Could you check a few things on this model? Use its own coordinates, in mm. Face numbers are marked on the shaded views. A direction names the side the tool comes from. Coordinates: 2 decimals unless noted, no trailing zeros. Write each loop counter-clockwise with the first axis right and the second up, starting at its lowest first coordinate (ties: lowest second). Pieces come first, ordered by that corner, then holes.
```python
from build123d import *

# Parameters (mm, degrees)
EXTRUDE_1_DEPTH        = 65
CUT_EXTRUDE_1_DEPTH    = 57.5
SKETCH_4_R             = 1.25
SKETCH_4_W             = 13
SKETCH_4_H             = 28.5
CUT_EXTRUDE_2_DEPTH    = 13
SKETCH_9_W             = 13
SKETCH_9_H             = 38.4
CUT_EXTRUDE_6_DEPTH    = 75.806476324
CUT_EXTRUDE_7_DEPTH    = 18
SKETCH_13_W            = 21
SKETCH_13_H            = 5
CUT_EXTRUDE_10_DEPTH   = 18
CUT_EXTRUDE_8_DEPTH    = 78.086308123
CUT_EXTRUDE_9_DEPTH    = 10
FILLET_1_R             = 4
FILLET_1_OF_MIRROR_3_R = 4
SKETCH_21_W            = 21
SKETCH_21_H            = 14
CUT_EXTRUDE_17_DEPTH   = 8
SKETCH_17_W            = 19.798748342
SKETCH_17_H            = 9
CUT_EXTRUDE_13_DEPTH   = 3
SKETCH_18_W            = 14
SKETCH_18_H            = 18
CUT_EXTRUDE_14_DEPTH   = 5
SKETCH_19_R            = 4
CUT_EXTRUDE_15_DEPTH   = 10
FILLET_6_R             = 2
SKETCH_5_R             = 12
CUT_EXTRUDE_3_DEPTH    = 8
CUT_EXTRUDE_16_DEPTH   = 61.954985592
CUT_EXTRUDE_18_DEPTH   = 25
CUT_EXTRUDE_19_DEPTH   = 20
CUT_EXTRUDE_5_DEPTH    = 76.706738594
CUT_EXTRUDE_20_DEPTH   = 12
FILLET_5_R             = 10


with BuildPart() as part:
    # 草圖1 → 填料-伸長1 (new body)
    with BuildSketch(Plane(origin=(0, 0, 0), x_dir=(1, 0, 0), z_dir=(0, 1, 0))):
        Polygon((0, 0), (24.34, 0), (34.67, -10.33), (34.67, -22.7), (-10.33, -22.7), (-10.33, -10.33), align=None)
    extrude(amount=EXTRUDE_1_DEPTH)

    # 草圖2 → 除料-伸長1 (cut)
    with BuildSketch(Plane(origin=(0, 5, 0), x_dir=(1, 0, 0), z_dir=(0, 1, 0))):
        Polygon((0, 0), (-22.7, -22.7), (-17.043145751, -22.7), (5.656854249, 0), align=None)
    cut_extrude_1 = extrude(amount=CUT_EXTRUDE_1_DEPTH, mode=Mode.SUBTRACT)

    # 鏡射1: 除料-伸長1 across plane
    add(cut_extrude_1.mirror(Plane.ZY.offset(-12.17)), mode=Mode.SUBTRACT)

    # 草圖4 → 除料-伸長2 (cut)
    with BuildSketch(Plane.XY.offset(22.7)):
        with Locations((12.17, 59.36)):
            Circle(SKETCH_4_R)
        with Locations((12.17, 24.36)):
            Circle(SKETCH_4_R)
        with Locations((12.17, 41.86)):
            Rectangle(SKETCH_4_W, SKETCH_4_H)
    extrude(amount=-CUT_EXTRUDE_2_DEPTH, mode=Mode.SUBTRACT)

    # 草圖9 → 除料-伸長6 (cut, through all)
    with BuildSketch(Plane.XY.offset(9.7)):
        with Locations((12.17, 41.86)):
            Rectangle(SKETCH_9_W, SKETCH_9_H)
    extrude(amount=-CUT_EXTRUDE_6_DEPTH, mode=Mode.SUBTRACT)

    # 草圖10 → 除料-伸長7 (cut)
    with BuildSketch(Plane.XZ):
        Polygon((20.67, 3), (3.67, 3), (1.67, 5), (1.67, 10), (22.67, 10), (22.67, 5), align=None)
    extrude(amount=-CUT_EXTRUDE_7_DEPTH, mode=Mode.SUBTRACT)

    # 草圖13 → 除料-伸長10 (cut)
    with BuildSketch(Plane.XZ):
        with Locations((12.17, 12.5)):
            Rectangle(SKETCH_13_W, SKETCH_13_H)
    extrude(amount=-CUT_EXTRUDE_10_DEPTH, mode=Mode.SUBTRACT)

    # 草圖11 → 除料-伸長8 (cut, through all)
    with BuildSketch(Plane.XZ):
        Polygon((-9.55794071, 4.584194914), (-25.114289896, 20.1405441), (-14.849242405, 30.405591591), (0.707106781, 14.849242405), align=None)
    cut_extrude_8 = extrude(amount=-CUT_EXTRUDE_8_DEPTH, mode=Mode.SUBTRACT)

    # 草圖12 → 除料-伸長9 (cut)
    with BuildSketch(Plane.XZ):
        Polygon((-4.242640687, 9.899494937), (-19.798989873, 25.455844123), (-11.313708499, 33.941125497), (4.242640687, 18.384776311), align=None)
    cut_extrude_9 = extrude(amount=-CUT_EXTRUDE_9_DEPTH, mode=Mode.SUBTRACT)

    # 圓角1
    fillet_1_edges = [part.edges().sort_by_distance(p)[0] for p in [
        (-3.218272016, 10, 18.774621202),
    ]]
    fillet(fillet_1_edges, radius=FILLET_1_R)

    # 鏡射3: 除料-伸長8, 除料-伸長9 across plane
    add(cut_extrude_8.mirror(Plane.ZY.offset(-12.17)), mode=Mode.SUBTRACT)
    add(cut_extrude_9.mirror(Plane.ZY.offset(-12.17)), mode=Mode.SUBTRACT)

    # 圓角1 of 鏡射3
    fillet_1_of_mirror_3_edges = [part.edges().sort_by_distance(p)[0] for p in [
        (27.558272016, 10, 18.774621202),
    ]]
    fillet(fillet_1_of_mirror_3_edges, radius=FILLET_1_OF_MIRROR_3_R)

    # 草圖21 → 除料-伸長17 (cut)
    with BuildSketch(Plane(origin=(0, 0, 0), x_dir=(-1, 0, 0), z_dir=(0, 0, -1))):
        with Locations((-12.17, 7)):
            Rectangle(SKETCH_21_W, SKETCH_21_H)
    extrude(amount=-CUT_EXTRUDE_17_DEPTH, mode=Mode.SUBTRACT)

    # 草圖17 → 除料-伸長13 (cut)
    with BuildSketch(Plane(origin=(2.828427125, 0, 2.828427125), x_dir=(-0.7071067811865472, 0, 0.7071067811865479), z_dir=(-0.7071067811865479, 0, -0.7071067811865472))):
        with Locations((11.537637522, 9.5)):
            Rectangle(SKETCH_17_W, SKETCH_17_H)
    extrude(amount=-CUT_EXTRUDE_13_DEPTH, mode=Mode.SUBTRACT)

    # 草圖18 → 除料-伸長14 (cut)
    with BuildSketch(Plane.XY.offset(15)):
        with Locations((12.17, 9)):
            Rectangle(SKETCH_18_W, SKETCH_18_H)
    extrude(amount=CUT_EXTRUDE_14_DEPTH, mode=Mode.SUBTRACT)

    # 草圖19 → 除料-伸長15 (cut)
    with BuildSketch(Plane.XY.offset(22.7)):
        with Locations((12.17, 24.36)):
            Circle(SKETCH_19_R)
    extrude(amount=-CUT_EXTRUDE_15_DEPTH, mode=Mode.SUBTRACT)

    # 圓角6
    fillet_6_edges = [part.edges().sort_by_distance(p)[0] for p in [
        (0.707106781, 39.5, 14.849242405),
        (3.889087297, 10, 18.03122292),
        (1.535533906, 11.171572875, 15.67766953),
        (23.632893219, 39.5, 14.849242405),
        (20.450912703, 10, 18.03122292),
        (22.804466094, 11.171572875, 15.67766953),
    ]]
    fillet(fillet_6_edges, radius=FILLET_6_R)

    # 草圖5 → 除料-伸長3 (cut)
    with BuildSketch(Plane.XY.offset(22.7)):
        with Locations((12.17, 50)):
            Circle(SKETCH_5_R)
    extrude(amount=-CUT_EXTRUDE_3_DEPTH, mode=Mode.SUBTRACT)

    # 草圖20 → 除料-伸長16 (cut, through all)
    with BuildSketch(Plane.XZ.offset(-18)):
        Polygon((4.17, 3.608174593), (-2.121320344, 9.899494937), (1.17918472, 13.2), (4.17, 13.2), align=None)
        Polygon((20.17, 13.2), (23.16081528, 13.2), (26.461320344, 9.899494937), (20.17, 3.608174593), align=None)
    extrude(amount=-CUT_EXTRUDE_16_DEPTH, mode=Mode.SUBTRACT)

    # 草圖22 → 除料-伸長18 (cut)
    with BuildSketch(Plane.XZ.offset(-14)):
        Polygon((1.414213562, 16.263455967), (-3.52233047, 21.2), (3.67, 21.2), (3.67, 18.519242405), align=None)
        Polygon((27.86233047, 21.2), (20.67, 21.2), (20.67, 18.519242405), (22.925786438, 16.263455967), align=None)
    extrude(amount=-CUT_EXTRUDE_18_DEPTH, mode=Mode.SUBTRACT)

    # 草圖23 → 除料-伸長19 (cut)
    with BuildSketch(Plane.XZ.offset(-18)):
        Polygon((4.17, 13.2), (1.17918472, 13.2), (4.17, 16.19081528), align=None)
        Polygon((23.16081528, 13.2), (20.17, 16.19081528), (20.17, 13.2), align=None)
    extrude(amount=-CUT_EXTRUDE_19_DEPTH, mode=Mode.SUBTRACT)

    # 草圖8 → 除料-伸長5 (cut, through all)
    with BuildSketch(Plane.XY.offset(22.7)):
        with BuildLine():
            Line((4.67, 70), (4.67, 73.83732793))
            Line((4.67, 73.83732793), (19.67, 73.83732793))
            Line((19.67, 73.83732793), (19.67, 70))
            ThreePointArc((19.67, 70), (12.17, 62.5), (4.67, 70))
        make_face()
    extrude(amount=-CUT_EXTRUDE_5_DEPTH, mode=Mode.SUBTRACT)

    # 草圖7 → 除料-伸長20 (cut)
    with BuildSketch(Plane.XY.offset(22.7)):
        with BuildLine():
            Line((-2.83, 70), (27.17, 70))
            ThreePointArc((27.17, 70), (12.17, 55), (-2.83, 70))
        make_face()
    extrude(amount=-CUT_EXTRUDE_20_DEPTH, mode=Mode.SUBTRACT)

    # 圓角5
    # the kernel refuses this fillet: 10 mm, written as the material it takes off along each edge
    with BuildSketch(Plane(origin=(3.203430143, 57.975, 14.7), x_dir=(-0.6822618553726185, 0.7311078994946726, 0), z_dir=(0, 0, 1))) as fillet_5_piece_1:
        with BuildLine():
            CenterArc((7.130730412, 9.839819243), FILLET_5_R, 209.862696675, 49.868396236)
            ThreePointArc((-1.541480723, 4.86058697), (-0.50958274, 2.5131167), (0, 0))
            ThreePointArc((0, 0), (2.674023904, 0.240271135), (5.348047809, 0))
        make_face()
    extrude(amount=21.370119522, mode=Mode.SUBTRACT)
    with BuildSketch(Plane(origin=(21.136569857, 57.975, 14.7), x_dir=(0.490653030896535, -0.8713550385876264, 0), z_dir=(0, 0, 1))) as fillet_5_piece_2:
        with BuildLine():
            CenterArc((7.223814974, 9.771686454), FILLET_5_R, 207.864748404, 49.868396236)
            ThreePointArc((-1.616718622, 5.097826622), (-0.579329834, 2.621547444), (0, 0))
            ThreePointArc((0, 0), (2.549581756, 0.273976255), (5.099163511, 0))
        make_face()
    extrude(amount=21.370119522, mode=Mode.SUBTRACT)


solid = part.part
```
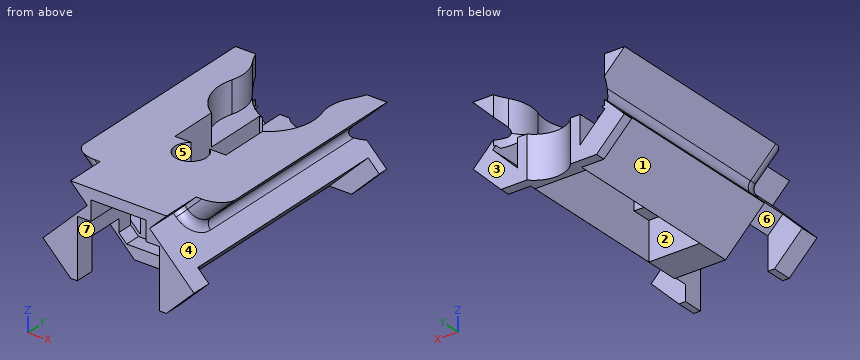
1. If we mould it in two halves opening along X, with no side actions, what happens to the marked faces 1, 2, 3 and 4? For each: pulls with the +X half, pulls with the -X half, needs draft (parallel to the pull), parting line crosses it, or undercut.
Verdict:
face 1: pulls with the -X half
face 2: undercut
face 3: needs draft
face 4: pulls with the +X half
2. I want a section at C-C on z = 1.75. Please give me the cut outline in (x, y), plus the area to 3 significant figures.
Verdict:
outline: (-1.75, 0) - (1.67, 0) - (1.67, 5) - (-1.75, 5) - close; (-1.75, 62.5) - (3.91, 62.5) - (3.91, 14) - (20.43, 14) - (20.43, 62.5) - (26.09, 62.5) - (26.09, 65) - (17.76, 65) arc R7.5 cw to (6.58, 65) - (-1.75, 65) - close; (22.67, 0) - (26.09, 0) - (26.09, 5) - (22.67, 5) - close; hole (5.67, 22.66) - (18.67, 22.66) - (18.67, 61.06) - (5.67, 61.06) - close
area: 387 mm2
3. For pin 1 (10 mm diameter, centred on y = 49, z = 7, fed in from -X); pin 2 (8.5 mm diameter, centred on x = 16.5, z = 10.5, fed in from -Y); pin 3 (1.5 mm diameter, centred on x = 0.5, z = 18.5, fed in from +Y), each with a flat end and sliding along its axis, tell me the tip position at first contact or that it passes through.
Verdict:
pin 1: stops at x = -4.24
pin 2: stops at y = 18
pin 3: stops at y = 61.57
4. I want a section at A-A on x = 12.17. Please give me the cut outline in (y, z), plus the area to 3 significant figures.
Verdict:
outline: (0, 20) - (18, 20) - (18, 3) - (14, 3) - (14, 0) - (22.66, 0) - (22.66, 9.7) - (23.11, 9.7) - (23.11, 12.7) - (20.36, 12.7) - (20.36, 22.7) - (0, 22.7) - close; (25.61, 9.7) - (27.61, 9.7) - (27.61, 12.7) - (25.61, 12.7) - close; (56.11, 9.7) - (58.11, 9.7) - (58.11, 10.7) - (56.11, 10.7) - close; (60.61, 9.7) - (61.06, 9.7) - (61.06, 0) - (62.5, 0) - (62.5, 10.7) - (60.61, 10.7) - close
area: 169 mm2
5. On a 3-axis mill with a long thin cutter (end or side, diameter ignored), from which of +Z, -Z, +X, -X, +Y, -Y can I reach the whole of each face in a straight line? I mean the marked faces 5, 6 and 7. Say none if no direction works.
Verdict:
face 5: +Z
face 6: -Z, -X
face 7: -Y
6. Please list where these lines run through material, in increasing order: line 1 along Y through (x, z) = (12.17, 10.6); line 2 along X through (y, z) = (37, 18.5); line 3 along Z through (x, y) = (27.5, 27).
Verdict:
line 1: y = 18 to 23.11, 25.61 to 27.61, 56.11 to 58.11, 60.61 to 62.5
line 2: x = -2.94 to -0.82, 3.65 to 5.67, 18.67 to 20.69, 25.16 to 27.28
line 3: z = 8.82 to 10.98, 18.72 to 20.84, 21.2 to 22.7
7. I want a section at B-B on y = 52. Give the number of separate pieces and of enclosed holes in the cut face, plus the area to 3 significant figures.
Verdict:
separate pieces: 2
enclosed holes: 2
area: 158 mm2
